Print and shaded views of the part. All mm, measured from the part's lowest x, y and z. A direction names the side the tool comes from. Round coordinates to 2 decimals unless told otherwise and drop trailing zeros. Write each loop counter-clockwise with the first axis right and the second up, starting at its lowest first coordinate (ties: lowest second). Pieces come first, ordered by that corner, then holes. Notation, with made-up numbers: (33.25, 26.25) -> (64.25, 26.25) arc R13 cw to (64.25, 34.25) -> close; hole circle Ø1 at (81, 67). An arc over 180 degrees is marked (long way). Return JSON: item names as keys, results as strings. Group by question number.
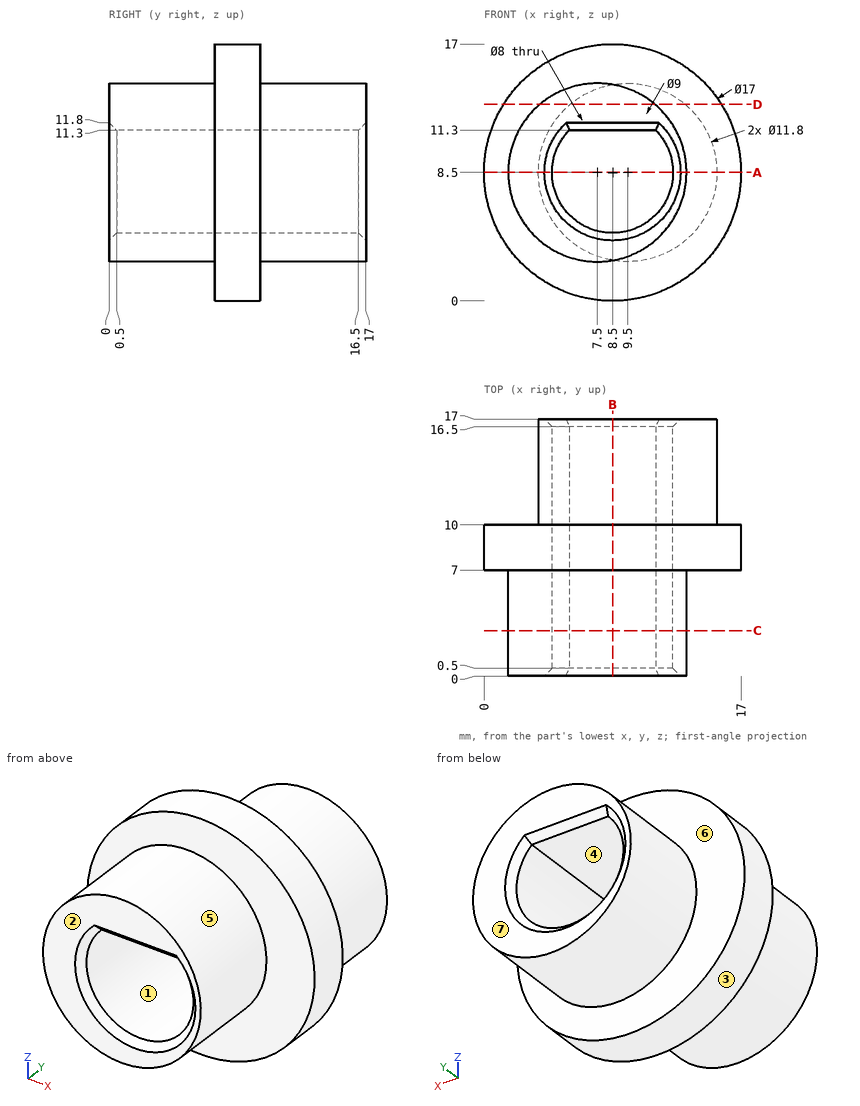
Item 1: Flat gauge pins, fed straight in: P1, Ø3, axis at y = 10.5, z = 13, coming from the +X side; P2, Ø1, axis at y = 4, z = 5.5, coming from the +X side; P3, Ø8, axis at x = 11.5, y = 2, coming from the +Z side. Where does each tip first touch, or does it go through?
Item 2: Cut at C-C (y = 3). Write the cut outline in (x, z).
Item 3: Cut at B-B (x = 8.5). Write the cut outline in (y, z).
Item 4: Cut at A-A (z = 8.5). Write the cut outline in (x, y).
Item 5: Which spindle directions (+Z, -Z, +X, -X, +Y, -Y) get a long thin tool onto all of the face, cutting with end or side? Do the marked faces 4, 5, 6 and 7. Say none if no direction does.
Item 6: Two-plate mould, pull along Z, no slides. Class the marked faces 1, 2 and 3: released by +Z, released by -Z, zero draft, split by the parting line, or undercut.
Item 7: Cut at D-D (z = 13). Write the cut outline in (x, y), then the cut area to 3 significant figures.
Item 8: Wall check: L1, parallel to X at y = 13.75, z = 8.5; L2, parallel to Y at x = 14.75, z = 5.75; L3, parallel to X at y = 5, z = 8.5. Give the ranges that are in metal, low to high.
Checks:
{
 "1": {"P1": "stops at x = 16.42", "P2": "stops at x = 12.84", "P3": "stops at z = 14.4"},
 "2": {"outline": "circle Ø11.8 at (7.5, 8.5); hole (5.64, 11.3) arc R4 ccw (long way) to (11.36, 11.3) -> close"},
 "3": {"outline": "(0, 2.69) -> (7, 2.69) -> (7, 0) -> (10, 0) -> (10, 2.69) -> (17, 2.69) -> (17, 4) -> (16.5, 4.5) -> (0.5, 4.5) -> (0, 4) -> close; (0, 11.8) -> (0.5, 11.3) -> (16.5, 11.3) -> (17, 11.8) -> (17, 14.31) -> (10, 14.31) -> (10, 17) -> (7, 17) -> (7, 14.31) -> (0, 14.31) -> close"},
 "4": {"outline": "(0, 7) -> (1.6, 7) -> (1.6, 0) -> (4, 0) -> (4.5, 0.5) -> (4.5, 16.5) -> (4, 17) -> (3.6, 17) -> (3.6, 10) -> (0, 10) -> close; (12.5, 0.5) -> (13, 0) -> (13.4, 0) -> (13.4, 7) -> (17, 7) -> (17, 10) -> (15.4, 10) -> (15.4, 17) -> (13, 17) -> (12.5, 16.5) -> close"},
 "5": {"face 4": "+Y, -Y", "face 5": "-Y", "face 6": "+Y", "face 7": "+Z, -Z, +X, -X, +Y"},
 "6": {"face 1": "undercut", "face 2": "zero draft", "face 3": "split by the parting line"},
 "7": {"outline": "(1.29, 7) -> (3.68, 7) -> (3.68, 0) -> (11.32, 0) -> (11.32, 7) -> (15.71, 7) -> (15.71, 10) -> (13.32, 10) -> (13.32, 17) -> (5.68, 17) -> (5.68, 10) -> (1.29, 10) -> close", "area": "150 mm2"},
 "8": {"L1": "x = 3.6 to 4.5, 12.5 to 15.4", "L2": "y = 7 to 10", "L3": "x = 1.6 to 4.5, 12.5 to 13.4"}
}
